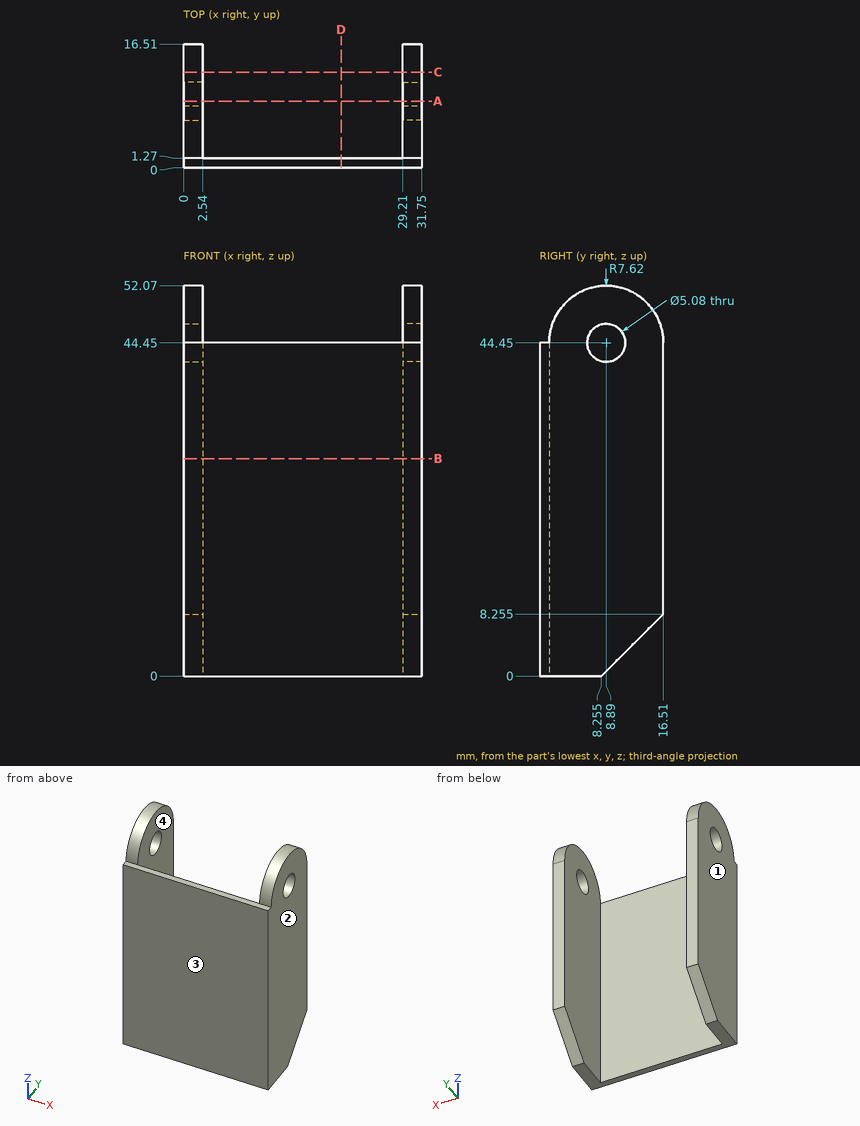
The drawing under review shows one solid part. Ordinate dimensions are in mm from its lowest x, y, z. Give positions to 0.01 mm unless a question says otherwise; leave off trailing zeros. Loops run counter-clockwise (first coordinate to the right, second up) from the corner with the lowest first, then second, coordinate; pieces in that order, holes last. Notation, with made-up numbers: M -19,40 L 9,40 A16 cw 9,68 Z; hole C -28.5,-26.5 d7. An arc over 180 degrees is marked long. One line per item, written item: value. Start each with the question number.
Q1. For L1, parallel to X at y = 5.75, z = 37; L2, parallel to Y at x = 28, z = 37; L3, parallel to Z at x = 1.3, y = 8.89 (3 decimals), list the stretches that pass through material, from the lowest coordinate up.
Q2. Clearance check with flat-ended pins moving along their axes: pin 1 Ø6 at (x, z) = (11, 31) entering from -Y; pin 2 Ø8 at (x, z) = (16, 24) entering from +Y; pin 3 Ø6 at (x, y) = (9.5, 7) entering from -Z. State where each tip first meets the part, or that it passes through.
Q3. Draft analysis for pull direction X (two halves, no side actions). For the marked faces 1, 2, 3 and 4, state which applies: released by +X, released by -X, zero draft, split by the parting line, or undercut.
Q4. Add section B-B (z = 29). Give the boundary of the cut face in (x, y), and give its area (3 significant figures).
Q5. Add section C-C (y = 12.75). Give the boundary of the cut face in (x, z) (3 decimals), and give its area (3 significant figures).
Q6. Add section A-A (y = 8.89). Give the boundary of the cut face in (x, z) (3 decimals).
Q7. Add section D-D (x = 21). Give the boundary of the cut face in (y, z).
Reply:
1. L1: 0 to 2.54, 29.21 to 31.75
1. L2: 0 to 1.27
1. L3: 0.635 to 41.91, 46.99 to 52.07
2. pin 1: y = 0
2. pin 2: y = 1.27
2. pin 3: through
3. face 1: released by -X
3. face 2: released by +X
3. face 3: zero draft
3. face 4: undercut
4. outline: M 0,0 L 31.75,0 L 31.75,16.51 L 29.21,16.51 L 29.21,1.27 L 2.54,1.27 L 2.54,16.51 L 0,16.51 Z
4. area: 118 mm²
5. outline: M 0,4.495 L 2.54,4.495 L 2.54,51.02 L 0,51.02 Z; M 29.21,4.495 L 31.75,4.495 L 31.75,51.02 L 29.21,51.02 Z
5. area: 236 mm²
6. outline: M 0,0.635 L 2.54,0.635 L 2.54,41.91 L 0,41.91 Z; M 0,46.99 L 2.54,46.99 L 2.54,52.07 L 0,52.07 Z; M 29.21,0.635 L 31.75,0.635 L 31.75,41.91 L 29.21,41.91 Z; M 29.21,46.99 L 31.75,46.99 L 31.75,52.07 L 29.21,52.07 Z
7. outline: M 0,0 L 1.27,0 L 1.27,44.45 L 0,44.45 Z
